CAD build for the part. Positions are in the model's coordinates, mm. A direction names the side the tool comes from. Coordinates: 2 decimals unless noted, no trailing zeros. Write each loop counter-clockwise with the first axis right and the second up, starting at its lowest first coordinate (ties: lowest second). Pieces come first, ordered by that corner, then holes. Notation, with made-up numbers: (36, 23.25) -> (71, 23.25) arc R26 ccw to (71, 58.25) -> close; hole circle Ø10 at (71, 0.5). An arc over 180 degrees is marked (long way). Answer as CSV lines item,"result".
```python
from build123d import *

# Parameters (mm, degrees)
SKETCH1_R           = 20
BOSS_EXTRUDE1_DEPTH = 30
BOSS_EXTRUDE2_DEPTH = 2
SKETCH3_R           = 1.55
SKETCH3_R_2         = 1.5
CUT_EXTRUDE1_DEPTH  = 2
FILLET1_R           = 1
FILLET2_R           = 10


with BuildPart() as part:
    # Sketch1 → Boss-Extrude1 (new body)
    with BuildSketch(Plane(origin=(0, 0, 0), x_dir=(1, 0, 0), z_dir=(0, 1, 0))):
        Circle(SKETCH1_R)
    extrude(amount=BOSS_EXTRUDE1_DEPTH)

    # Sketch2 → Boss-Extrude2 (add)
    with BuildSketch(Plane.XZ):
        with BuildLine():
            Line((-9, 46), (-9, 17.860571099))
            ThreePointArc((-9, 17.860571099), (0, 20), (9, 17.860571099))
            Line((9, 17.860571099), (9, 46))
            Line((9, 46), (-9, 46))
        make_face()
    extrude(amount=-BOSS_EXTRUDE2_DEPTH)

    # Sketch3 → Cut-Extrude1 (cut)
    with BuildSketch(Plane(origin=(0, 2, 0), x_dir=(1, 0, 0), z_dir=(0, 1, 0))):
        with Locations((-1, -40)):
            Circle(SKETCH3_R)
        with Locations((0, -23.5)):
            Circle(SKETCH3_R_2)
    extrude(amount=-CUT_EXTRUDE1_DEPTH, mode=Mode.SUBTRACT)

    # Fillet1
    fillet1_edges = [part.edges().sort_by_distance(p)[0] for p in [
        (-9, 1, 17.860571099),
        (0, 2, 20),
        (9, 1, 17.860571099),
    ]]
    fillet(fillet1_edges, radius=FILLET1_R)

    # Fillet2
    fillet2_edges = [part.edges().sort_by_distance(p)[0] for p in [
        (-20, 30, 0),
    ]]
    fillet(fillet2_edges, radius=FILLET2_R)


solid = part.part
```
Item 1: Flat gauge pins, fed straight in: pin 1 (1.5 mm diameter, centred on x = -10.5, y = 17.5, fed in from -Z); pin 2 (8 mm diameter, centred on y = 20.5, z = 15.5, fed in from -X); pin 3 (3 mm diameter, centred on y = 11, z = 8.5, fed in from +X) (3 decimals). Where does each tip first touch, or does it go through?
Answer below:
pin 1,"stops at z = -17.46"
pin 2,"stops at x = -16.35"
pin 3,"stops at x = 18.735"
Item 2: Saw through at A-A on z = 23.5. Give the cut face in (x, y).
Answer below:
outline,"(-9, 0) -> (-1.5, 0) -> (-1.5, 2) -> (-9, 2) -> close; (1.5, 0) -> (9, 0) -> (9, 2) -> (1.5, 2) -> close"
Item 3: Saw through at C-C on y = 11.5. Give the cut face in (x, z).
Answer below:
outline,"circle Ø40 at (0, 0)"
Item 4: Wall check: line 1 (X direction, y = 1.4, z = 40); line 2 (X direction, y = 0.6, z = 23.5); line 3 (Z direction, x = 0, y = 1). Give the ranges that are in metal, low to high. Write a range as from..to.
Answer below:
line 1,"x = -9..-2.55, 0.55..9"
line 2,"x = -9..-1.5, 1.5..9"
line 3,"z = -20..22, 25..38.82, 41.18..46"
Item 5: Saw through at B-B on z = 40. Give the cut face in (x, y).
Answer below:
outline,"(-9, 0) -> (-2.55, 0) -> (-2.55, 2) -> (-9, 2) -> close; (0.55, 0) -> (9, 0) -> (9, 2) -> (0.55, 2) -> close"
Item 6: Two-plate mould, pull along Z, no slides. Class faces 6 (the flat face through (0, 1, 46)), 7 (the flat face through (0, 2, 33)), 8 (the cylindrical face through (0, 1, 22)): pulls with the +Z half, pulls with the -Z half, needs draft (parallel to the pull), parting line crosses it, or undercut.
Answer below:
face 6,"pulls with the +Z half"
face 7,"needs draft"
face 8,"undercut"
Item 7: 3-axis set-ups, long thin cutter, end or side, ignore diameter. For faces 1 (the flat face through (9, 1, 32)), 2 (the flat face through (0, 0, 5)), 3 (the flat face through (0, 30, 0)), 4 (the cylindrical face through (-2.6, 9.86, -19.83)), 5 (the flat face through (-9, 1, 32)): which of +Z, -Z, +X, -X, +Y, -Y reach the whole face in a straight line?
Answer below:
face 1,"+Z, +X, +Y, -Y"
face 2,"+Z, -Z, +X, -X, -Y"
face 3,"+Z, -Z, +X, -X, +Y"
face 4,"+Y"
face 5,"+Z, -X, +Y, -Y"
